```python
from build123d import *

# Parameters (mm, degrees)
IZIM1_W                     = 85
IZIM1_H                     = 85
Y_KSEKLIK_EKSTR_ZYON1_DEPTH = 5
IZIM2_R                     = 32.5
KES_EKSTR_ZYON1_DEPTH       = 5
IZIM3_R                     = 42.5
IZIM3_R_2                   = 38
Y_KSEKLIK_EKSTR_ZYON2_DEPTH = 25
IZIM4_R                     = 2
KES_EKSTR_ZYON2_DEPTH       = 25


with BuildPart() as part:
    # Çizim1 → Yükseklik-Ekstrüzyon1 (new body)
    with BuildSketch(Plane(origin=(0, 0, 0), x_dir=(1, 0, 0), z_dir=(0, 1, 0))):
        Rectangle(IZIM1_W, IZIM1_H)
    extrude(amount=Y_KSEKLIK_EKSTR_ZYON1_DEPTH)

    # Çizim2 → Kes-Ekstrüzyon1 (cut)
    with BuildSketch(Plane(origin=(0, 5, 0), x_dir=(1, 0, 0), z_dir=(0, 1, 0))):
        with Locations(Location((0, 0, 0), (0, 0, 270))):
            Circle(IZIM2_R)
    extrude(amount=-KES_EKSTR_ZYON1_DEPTH, mode=Mode.SUBTRACT)

    # Çizim3 → Yükseklik-Ekstrüzyon2 (add)
    with BuildSketch(Plane(origin=(0, 5, 0), x_dir=(1, 0, 0), z_dir=(0, 1, 0))):
        with Locations(Location((0, 0, 0), (0, 0, 270))):
            Circle(IZIM3_R)
        with Locations(Location((0, 0, 0), (0, 0, 270))):
            Circle(IZIM3_R_2, mode=Mode.SUBTRACT)
    extrude(amount=Y_KSEKLIK_EKSTR_ZYON2_DEPTH)

    # Çizim4 → Kes-Ekstrüzyon2 (cut)
    with BuildSketch(Plane(origin=(0, 5, 0), x_dir=(1, 0, 0), z_dir=(0, 1, 0))):
        with Locations(Location((-34.943063938, 32.5, 0), (0, 0, 270))):
            Circle(IZIM4_R)
        with Locations(Location((32.5, 34.943063938, 0), (0, 0, 270))):
            Circle(IZIM4_R)
        with Locations(Location((34.943063938, -32.5, 0), (0, 0, 270))):
            Circle(IZIM4_R)
        with Locations(Location((-32.5, -34.943063938, 0), (0, 0, 270))):
            Circle(IZIM4_R)
    extrude(amount=-KES_EKSTR_ZYON2_DEPTH, mode=Mode.SUBTRACT)


solid = part.part
```
For this review, take the finished solid that the model builds, in its own axes (mm). A direction names the side the tool comes from. Give positions to 0.01 mm unless a question says otherwise; leave off trailing zeros. Write each loop counter-clockwise with the first axis right and the second up, starting at its lowest first coordinate (ties: lowest second). Pieces come first, ordered by that corner, then holes.
Item 1: Take a section at C-C (y = 9). Give the boundary of the cut face in (x, z), and give its area (3 significant figures).
Item 2: Take a section at B-B (x = 23). Give the boundary of the cut face in (y, z).
Item 3: Wall thickness on probe 1 along X at (y, z) = (2.25, 0); probe 2 along Z at (x, y) = (-34, 17); probe 3 along X at (y, z) = (15.5, 24.5): over which ranges is each line inside the solid? List them lowest first.
Item 4: The part is to be moulded in two halves that separate along X. For faces 1 (the face through (34.18, 2.54, 34.35)), 2 (the face through (-25.861, 17.325, -33.727)), 3 (the face through (-29, 0, 18)), say which applies: +X half, -X half, draft (parallel to the pull), parting line (faces both ways), or undercut.
Item 5: Take a section at A-A (z = 4). Give the boundary of the cut face in (x, y), and give its area (3 significant figures).
Item 6: Insertion check: P1, Ø1, axis at x = -17, y = 9, coming from the -Z side; P2, Ø4.5, axis at x = 32.5, z = -34.94, coming from the +Y side; P3, Ø1, axis at x = -22, y = 22, coming from the -Z side. Each pin has a flat end and moves straight along its axis. Give the tip position at first contact, or say it passes through.
Item 7: Machinability: for faces 4 (the face through (-36, 5, 34)), 5 (the face through (28, 5, -17)), 6 (the face through (-32, 5, -34)), 7 (the face through (32, 5, 34)), which of the approach directions +Z, -Z, +X, -X, +Y, -Y give a long, thin tool a straight path to every point of the face, cutting with its end or side? Answer none if there is none.
Established:
1. outline: circle Ø85 at (0, 0); hole circle Ø76 at (0, 0)
1. area: 1,140 mm2
2. outline: (0, -42.5) - (5, -42.5) - (5, -35.74) - (30, -35.74) - (30, -30.25) - (5, -30.25) - (5, -22.96) - (0, -22.96) - close; (0, 22.96) - (5, 22.96) - (5, 30.25) - (30, 30.25) - (30, 35.74) - (5, 35.74) - (5, 42.5) - (0, 42.5) - close
3. probe 1: x = -42.5 to -32.5, 32.5 to 42.5
3. probe 2: z = -25.5 to -16.97, 16.97 to 25.5
3. probe 3: x = -34.73 to -29.05, 29.05 to 34.73
4. face 1: undercut
4. face 2: parting line
4. face 3: draft
5. outline: (-42.5, 0) - (-32.25, 0) - (-32.25, 5) - (-37.79, 5) - (-37.79, 30) - (-42.31, 30) - (-42.31, 5) - (-42.5, 5) - close; (32.25, 0) - (42.5, 0) - (42.5, 5) - (42.31, 5) - (42.31, 30) - (37.79, 30) - (37.79, 5) - (32.25, 5) - close
5. area: 329 mm2
6. P1: stops at z = -39.17
6. P2: stops at y = 5
6. P3: stops at z = -36.66
7. face 4: +Z, -X, +Y
7. face 5: +Y
7. face 6: -Z, -X, +Y
7. face 7: +Z, +X, +Y
